from build123d import *

# Parameters (mm, degrees)
SKETCH1_W               = 69.85
SKETCH1_H               = 19.05
BOSS_EXTRUDE1_DEPTH     = 6.223
SKETCH4_W               = 25.4
SKETCH4_H               = 19.05
BOSS_EXTRUDE2_DEPTH     = 3.302
F_1_4_CLEARANCE_HOLE2_D = 6.7564


with BuildPart() as part:
    # Sketch1 → Boss-Extrude1 (new body)
    with BuildSketch(Plane(origin=(0, 0, 0), x_dir=(1, 0, 0), z_dir=(0, 1, 0))):
        Rectangle(SKETCH1_W, SKETCH1_H)
    extrude(amount=BOSS_EXTRUDE1_DEPTH)

    # Sketch4 → Boss-Extrude2 (add)
    with BuildSketch(Plane(origin=(0, 6.223, 0), x_dir=(1, 0, 0), z_dir=(0, 1, 0))):
        with Locations((22.225, 0)):
            Rectangle(SKETCH4_W, SKETCH4_H)
    extrude(amount=BOSS_EXTRUDE2_DEPTH)

    # 1/4 Clearance Hole2 (through all)
    with Locations(Plane(origin=(0, 0, 0), x_dir=(-1, 0, 0), z_dir=(0, -1, 0))):
        with Locations((-24.765, 0), (6.985, 0), (26.035, 0)):
            Hole(F_1_4_CLEARANCE_HOLE2_D / 2)


solid = part.part
The listing builds one solid part. Answer for the finished solid, in the listing's coordinates (mm). A direction names the side the tool comes from. Coordinates: 2 decimals unless noted, no trailing zeros. Write each loop counter-clockwise with the first axis right and the second up, starting at its lowest first coordinate (ties: lowest second). Pieces come first, ordered by that corner, then holes. Notation, with made-up numbers: (64.5, 56.25) -> (109.5, 56.25) arc R20 ccw to (109.5, 87.25) -> close; hole circle Ø10 at (27, 38). An arc over 180 degrees is marked (long way). One line per question, with ' | ' between items.
1. Straight lines are drawn through the part: line 1 (X direction, y = 9.25, z = 4) (3 decimals); line 2 (Y direction, x = -10.5, z = -4.75); line 3 (X direction, y = 8.25, z = -3) (3 decimals). For each, find the intervals that lie inside material, in ascending order.
Verdict:
line 1: x = 9.525 to 34.925 | line 2: y = 0 to 6.22 | line 3: x = 9.525 to 23.212, 26.318 to 34.925
2. For a pull along Z with two mould halves and no side action, classify faces 3 (the cylindrical face through (21.39, 4.83, -0.15)), 4 (the flat face through (0, 4, 9.525)), 5 (the flat face through (-34.925, 3, 0)) as released by +Z, released by -Z, zero draft, split by the parting line, or undercut.
Verdict:
face 3: undercut | face 4: released by +Z | face 5: zero draft
3. Section C-C (x = -26) is taken. Determine the outline of the cut face in (y, z) (3 decimals).
Verdict:
outline: (0, -9.525) -> (6.223, -9.525) -> (6.223, -3.378) -> (0, -3.378) -> close; (0, 3.378) -> (6.223, 3.378) -> (6.223, 9.525) -> (0, 9.525) -> close
4. Section B-B (y = 2) is taken. Determine the outline of the cut face in (x, z) (3 decimals), and give its area (3 significant figures).
Verdict:
outline: (-34.925, -9.525) -> (34.925, -9.525) -> (34.925, 9.525) -> (-34.925, 9.525) -> close; hole circle Ø6.756 at (-26.035, 0); hole circle Ø6.756 at (-6.985, 0); hole circle Ø6.756 at (24.765, 0) | area: 1,220 mm^2
5. Section D-D (z = -6.5) is taken. Determine the outline of the cut face in (x, y) (3 decimals), and give its area (3 significant figures).
Verdict:
outline: (-34.925, 0) -> (34.925, 0) -> (34.925, 9.525) -> (9.525, 9.525) -> (9.525, 6.223) -> (-34.925, 6.223) -> close | area: 519 mm^2
6. Which of the six approach directions +Z, -Z, +X, -X, +Y, -Y give full straight-line access (tool end or side, diameter ignored) to faces 1 (the flat face through (9.525, 8, 0)), 2 (the flat face through (0, 4, -9.525))?
Verdict:
face 1: +Z, -Z, -X, +Y | face 2: -Z, +X, -X, +Y, -Y
7. Section A-A (z = 0) is taken. Determine the outline of the cut face in (x, y) (3 decimals).
Verdict:
outline: (-34.925, 0) -> (-29.413, 0) -> (-29.413, 6.223) -> (-34.925, 6.223) -> close; (-22.657, 0) -> (-10.363, 0) -> (-10.363, 6.223) -> (-22.657, 6.223) -> close; (-3.607, 0) -> (21.387, 0) -> (21.387, 9.525) -> (9.525, 9.525) -> (9.525, 6.223) -> (-3.607, 6.223) -> close; (28.143, 0) -> (34.925, 0) -> (34.925, 9.525) -> (28.143, 9.525) -> close
8. Given pin 1 Ø4 at (x, z) = (-6.985, 0) entering from -Y; pin 2 Ø3.5 at (y, z) = (8.5, -2) entering from -X (3 decimals); pin 3 Ø9.5 at (x, z) = (-8.5, -1) entering from +Y, each flat-ended and moving along its own axis, determine where each tip first touches the part or whether it passes through.
Verdict:
pin 1: passes through | pin 2: stops at x = 9.525 | pin 3: stops at y = 6.22
